The listing builds one solid part. Answer for the finished solid, in the listing's coordinates (mm). Face numbers are marked on the shaded views. Round coordinates to 2 decimals unless told otherwise and drop trailing zeros. Order: outer loops, then holes, each group sorted by start corner. A loop starts at its lowest first (then second) coordinate and runs counter-clockwise, first axis right, second up. Notation, with made-up numbers: (64.5, -26) - (89.5, -26) arc R17 ccw to (89.5, -12) - close; hole circle Ø9 at (74.5, 62). An arc over 180 degrees is marked (long way). Use CSV: the item, a comma, the result in double quotes. Start each with the question number.
Item 1: Find section B-B, the plane x = 18. Give the vertices of the cut face in (y, z).
Item 2: Straight lines are drawn through the part: line 1 along X through (y, z) = (0, 206); line 2 along X through (y, z) = (31, 137.5). For each, find the intervals that lie inside material, in ascending order. Write a range as [from, to].
Item 3: Find section A-A, the plane z = 46. Give the vertices of the cut face in (x, y), plus the area to 3 significant figures.
Item 4: Find section C-C, the plane y = -21. Give the vertices of the cut face in (x, z).
Item 5: Find section D-D, the plane z = 179. Give the vertices of the cut face in (x, y), plus the area to 3 significant figures.
Item 6: Flat-ended cylindrical pins translate along their axes: P1, Ø8, axis at y = -7, z = 112, coming from the +X side; P2, Ø12, axis at x = -27.5, z = 228.5, coming from the +Y side; P3, Ø5, axis at y = 15.5, z = 199.5, coming from the -X side. Find the tip coordinate at first contact, or state that the pin passes through.
Item 7: Determine the mould class of the marked faces 1 and 2 for opening direction X: +X half, -X half, draft (parallel to the pull), parting line (faces both ways), or undercut.
Solid Edge part; units mm, degrees
sketch "Sketch1" plane through (0, 0, 0) normal (0, 0, 1) x (1, 0, 0)
  circle A0 centre (0, 0) radius 38.1
  circle A1 centre (0, 0) radius 37.211
extrude "Protrusion1" add sketch "Sketch1" along normal blind 304.8
sketch "Sketch2" plane through (-38.1, 0, 152.4) normal (-1, 0, 0) x (0, 0, -1)
  line L0 (88.9, 1.5875) -> (88.9, -1.5875)
  line L1 (88.9, -1.5875) -> (139.7, -1.5875)
  line L2 (139.7, -1.5875) -> (139.7, 1.5875)
  line L3 (139.7, 1.5875) -> (88.9, 1.5875)
extrude "ExtrudedCutout_1" cut sketch "Sketch2" against normal blind 12.7
pattern_circular "Pattern1" count 4 over 360 about axis through (0, 0, 0) along (0, 0, -1) of "ExtrudedCutout_1"
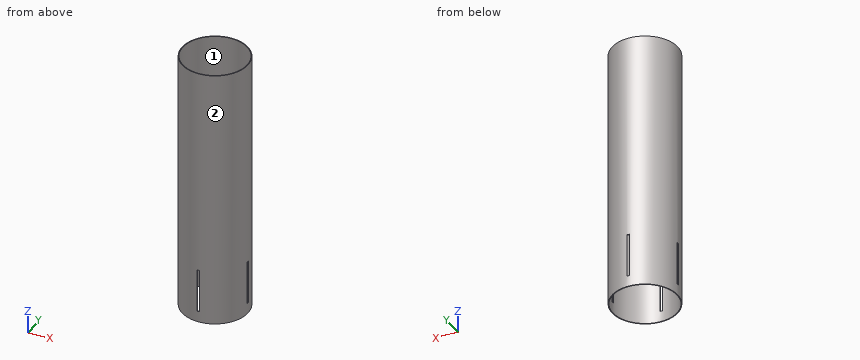
Worked out:
1,outline,"(-33.58, 0) - (-32.57, 0) - (-32.57, 304.8) - (-33.58, 304.8) - close; (32.57, 0) - (33.58, 0) - (33.58, 304.8) - (32.57, 304.8) - close"
2,line 1,"x = [-38.1, -37.21], [37.21, 38.1]"
2,line 2,"x = [-22.15, -20.58], [20.58, 22.15]"
3,outline,"(-38.07, -1.59) arc R38.1 ccw to (-1.59, -38.07) - (-1.59, -37.18) arc R37.21 cw to (-37.18, -1.59) - close; (-38.07, 1.59) - (-37.18, 1.59) arc R37.21 cw to (-1.59, 37.18) - (-1.59, 38.07) arc R38.1 ccw to start; (1.59, -38.07) arc R38.1 ccw to (38.07, -1.59) - (37.18, -1.59) arc R37.21 cw to (1.59, -37.18) - close; (1.59, 37.18) arc R37.21 cw to (37.18, 1.59) - (38.07, 1.59) arc R38.1 ccw to (1.59, 38.07) - close"
3,area,"199 mm²"
4,outline,"(-31.79, 0) - (-30.72, 0) - (-30.72, 304.8) - (-31.79, 304.8) - close; (30.72, 0) - (31.79, 0) - (31.79, 304.8) - (30.72, 304.8) - close"
5,outline,"circle Ø76.2 at (0, 0); hole circle Ø74.42 at (0, 0)"
5,area,"210 mm²"
6,P1,"stops at x = 37.98"
6,P2,"stops at y = 31.45"
6,P3,"stops at x = -35.81"
7,face 1,"undercut"
7,face 2,"parting line"
